The drawing under review shows one solid part. Ordinate dimensions are in mm from its lowest x, y, z. Give positions to 0.01 mm unless a question says otherwise; leave off trailing zeros. Loops run counter-clockwise (first coordinate to the right, second up) from the corner with the lowest first, then second, coordinate; pieces in that order, holes last. Notation, with made-up numbers: (10, 77.5) -> (35, 77.5) arc R13 ccw to (35, 83.5) -> close; hole circle Ø4 at (20.25, 59). An arc over 180 degrees is marked (long way). Answer in a Markdown table with one row per item. Add a question column.
(1) For line 1 (Y direction, x = 3.1, z = 2); line 2 (X direction, y = 70, z = 2.15) (1 decimal); line 3 (Y direction, x = 1.75, z = 2.3) (1 decimal), list the stretches that pass through material, from the lowest coordinate up.
(2) Consider section D-D on y = 41. Write out the cut boundary in (x, z) (1 decimal).
(3) Consider section A-A on z = 2. Write out the cut boundary in (x, y), then the cut area to 3 significant figures.
(4) For pin 1 (1.5 mm diameter, centred on x = 1, y = 38.5, fed in from +Z) (1 decimal); pin 2 (1 mm diameter, centred on x = 3.5, y = 57, fed in from -Z), all flat-tipped, find the tip position at first contact; note any pin that passes through.
(5) Consider section B-B on x = 0.8. Write out the cut boundary in (y, z).
(6) Consider section C-C on y = 72. Write out the cut boundary in (x, z), then the cut area to 3 significant figures.
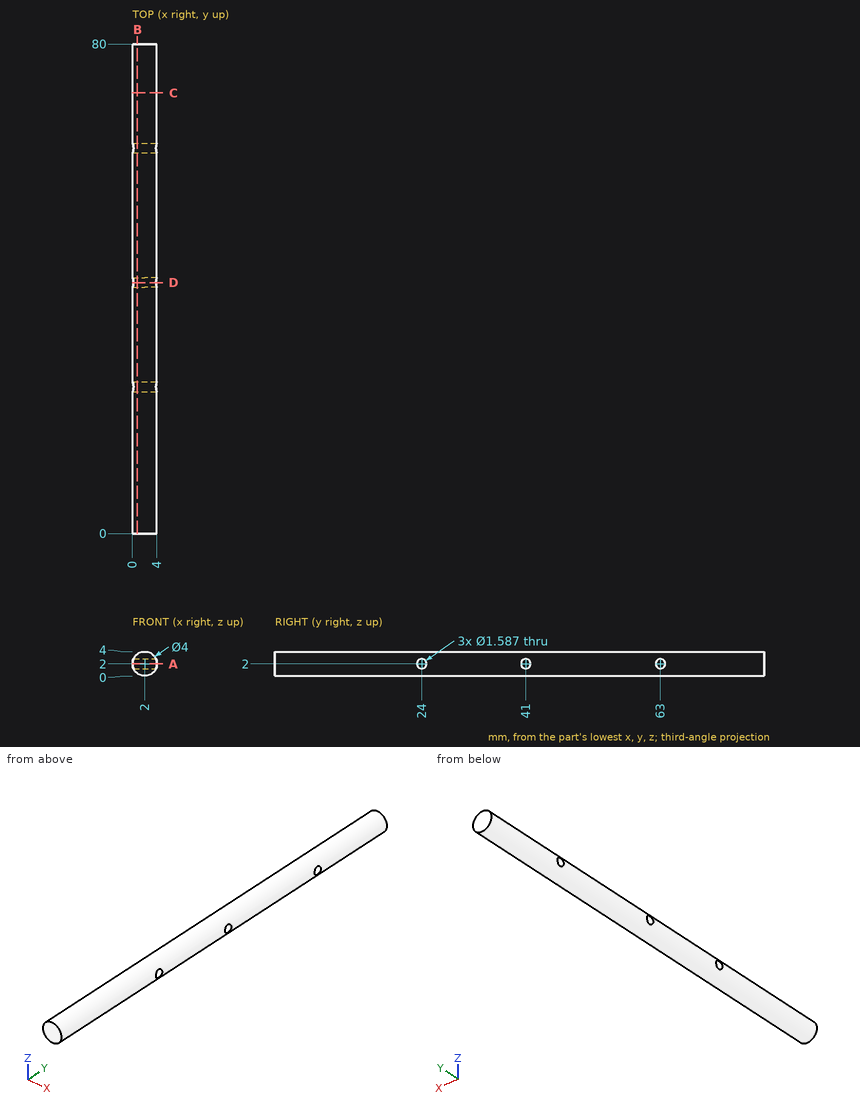
Values follow:
| question | item | result |
|---|---|---|
| 1 | line 1 | 0 to 23.21, 24.79 to 40.21, 41.79 to 62.21, 63.79 to 80 |
| 1 | line 2 | 0 to 4 |
| 1 | line 3 | 0 to 23.3, 24.7 to 40.3, 41.7 to 62.3, 63.7 to 80 |
| 2 | outline | (0.2, 1.2) arc R2 ccw to (3.8, 1.2) -> close; (0.2, 2.8) -> (3.8, 2.8) arc R2 ccw to start |
| 3 | outline | (0, 0) -> (4, 0) -> (4, 23.21) -> (0, 23.21) -> close; (0, 24.79) -> (4, 24.79) -> (4, 40.21) -> (0, 40.21) -> close; (0, 41.79) -> (4, 41.79) -> (4, 62.21) -> (0, 62.21) -> close; (0, 63.79) -> (4, 63.79) -> (4, 80) -> (0, 80) -> close |
| 3 | area | 301 mm2 |
| 4 | pin 1 | z = 4 |
| 4 | pin 2 | z = 0.27 |
| 5 | outline | (0, 0.4) -> (80, 0.4) -> (80, 3.6) -> (0, 3.6) -> close; hole circle Ø1.59 at (24, 2); hole circle Ø1.59 at (41, 2); hole circle Ø1.59 at (63, 2) |
| 6 | outline | circle Ø4 at (2, 2) |
| 6 | area | 12.6 mm2 |
